from build123d import *

# Parameters (mm, degrees)
SKETCH1_W                 = 12
SKETCH1_H                 = 25
BOSS_EXTRUDE1_DEPTH       = 16
SKETCH2_W                 = 32
SKETCH2_H                 = 10
BOSS_EXTRUDE2_DEPTH       = 16.2
BOSS_EXTRUDE3_DEPTH       = 32
M5X0_8_TAPPED_HOLE1_D     = 4.2
M5X0_8_TAPPED_HOLE1_DEPTH = 9
M5X0_8_TAPPED_HOLE1_TIP   = 1.2618073
CUT_EXTRUDE2_REACH        = 27
M3X0_5_TAPPED_HOLE1_D     = 2.75
M3X0_5_TAPPED_HOLE1_DEPTH = 12
M3X0_5_TAPPED_HOLE1_TIP   = 0.826183351


with BuildPart() as part:
    # Sketch1 → Boss-Extrude1 (new body, symmetric)
    with BuildSketch(Plane(origin=(0, 0, 0), x_dir=(0, 0, -1), z_dir=(1, 0, 0))):
        with Locations((6, 12.5)):
            Rectangle(SKETCH1_W, SKETCH1_H)
    extrude(amount=BOSS_EXTRUDE1_DEPTH, both=True)



with BuildPart() as body_2:
    # Sketch2 → Boss-Extrude2 (new body)
    with BuildSketch(Plane(origin=(0, 0, 0), x_dir=(1, 0, 0), z_dir=(0, 1, 0))):
        with Locations((0, -7)):
            Rectangle(SKETCH2_W, SKETCH2_H)
    extrude(amount=BOSS_EXTRUDE2_DEPTH)


with BuildPart() as part_1:
    add(part.part)

    add(body_2.part)  # Boss-Extrude3 merges body 2
    # Sketch3 → Boss-Extrude3 (add)
    with BuildSketch(Plane(origin=(16, 0, 0), x_dir=(0, 0, -1), z_dir=(1, 0, 0))):
        Polygon((-2, 0), (-2, 16.2), (0, 25), (0, 0), align=None)
    extrude(amount=-BOSS_EXTRUDE3_DEPTH)

    # M5x0.8 Tapped Hole1
    with Locations(Plane(origin=(0, 0, -12), x_dir=(-1, 0, 0), z_dir=(0, 0, -1))):
        with Locations((0, 20), (0, 5)):
            Hole(M5X0_8_TAPPED_HOLE1_D / 2, depth=M5X0_8_TAPPED_HOLE1_DEPTH)
            with Locations((0, 0, -(M5X0_8_TAPPED_HOLE1_DEPTH + M5X0_8_TAPPED_HOLE1_TIP / 2))):  # 118° drill point
                Cone(0, M5X0_8_TAPPED_HOLE1_D / 2, M5X0_8_TAPPED_HOLE1_TIP, mode=Mode.SUBTRACT)

    # Sketch9 → Cut-Revolve1 (revolve, cut)
    with BuildSketch(Plane(origin=(0, 0, 0), x_dir=(0, 0, -1), z_dir=(1, 0, 0))):
        Polygon((-12, 16.2), (-4, 16.2), (-4, 12), (-6, 12), (-6, 6.5), (-4, 6.5), (-4, 0), (-12, 0), align=None)
    revolve(axis=Axis((0, 0, 12), (0, 1, 0)), mode=Mode.SUBTRACT)

    # Sketch10 → Cut-Extrude2 (cut, up to next)
    with BuildSketch(Plane(origin=(0, 25, 0), x_dir=(1, 0, 0), z_dir=(0, 1, 0)), mode=Mode.PRIVATE) as cut_extrude2_sk1:
        Polygon((6.3625, 12), (14.623214286, 0), (16, 0), (16, 12), align=None)
    cut_extrude2_tool1 = extrude(cut_extrude2_sk1.sketch, amount=-CUT_EXTRUDE2_REACH, mode=Mode.PRIVATE) & part_1.part
    add(cut_extrude2_tool1.solids().sort_by_distance((12.730134, 25, -7.5))[0], mode=Mode.SUBTRACT)
    # Sketch10 → Cut-Extrude2 (cut, up to next)
    with BuildSketch(Plane(origin=(0, 25, 0), x_dir=(1, 0, 0), z_dir=(0, 1, 0)), mode=Mode.PRIVATE) as cut_extrude2_sk2:
        Polygon((16, 0), (14.623214286, 0), (16, -2), align=None)
    cut_extrude2_tool2 = extrude(cut_extrude2_sk2.sketch, amount=-CUT_EXTRUDE2_REACH, mode=Mode.PRIVATE) & part_1.part
    add(cut_extrude2_tool2.solids().sort_by_distance((15.541071, 25, 0.666667))[0], mode=Mode.SUBTRACT)
    # Sketch10 → Cut-Extrude2 (cut, up to next)
    with BuildSketch(Plane(origin=(0, 25, 0), x_dir=(1, 0, 0), z_dir=(0, 1, 0)), mode=Mode.PRIVATE) as cut_extrude2_sk3:
        Polygon((-16, 0), (-14.623214286, 0), (-6.3625, 12), (-16, 12), align=None)
    cut_extrude2_tool3 = extrude(cut_extrude2_sk3.sketch, amount=-CUT_EXTRUDE2_REACH, mode=Mode.PRIVATE) & part_1.part
    add(cut_extrude2_tool3.solids().sort_by_distance((-12.730134, 25, -7.5))[0], mode=Mode.SUBTRACT)
    # Sketch10 → Cut-Extrude2 (cut, up to next)
    with BuildSketch(Plane(origin=(0, 25, 0), x_dir=(1, 0, 0), z_dir=(0, 1, 0)), mode=Mode.PRIVATE) as cut_extrude2_sk4:
        Polygon((-16, 0), (-16, -2), (-14.623214286, 0), align=None)
    cut_extrude2_tool4 = extrude(cut_extrude2_sk4.sketch, amount=-CUT_EXTRUDE2_REACH, mode=Mode.PRIVATE) & part_1.part
    add(cut_extrude2_tool4.solids().sort_by_distance((-15.541071, 25, 0.666667))[0], mode=Mode.SUBTRACT)

    # M3x0.5 Tapped Hole1
    with Locations(Plane.XY.offset(12)):
        with Locations((-11.5, 13.25), (11.5, 13.25), (-11.5, 5.25), (11.5, 5.25)):
            Hole(M3X0_5_TAPPED_HOLE1_D / 2, depth=M3X0_5_TAPPED_HOLE1_DEPTH)
            with Locations((0, 0, -(M3X0_5_TAPPED_HOLE1_DEPTH + M3X0_5_TAPPED_HOLE1_TIP / 2))):  # 118° drill point
                Cone(0, M3X0_5_TAPPED_HOLE1_D / 2, M3X0_5_TAPPED_HOLE1_TIP, mode=Mode.SUBTRACT)


solid = part_1.part
Model file for the job. Use its own axes, mm. A direction names the side the tool comes from. Give positions to 0.01 mm unless a question says otherwise; leave off trailing zeros. Loops run counter-clockwise (first coordinate to the right, second up) from the corner with the lowest first, then second, coordinate; pieces in that order, holes last. Notation, with made-up numbers: (81, 82.5) -> (109, 82.5) arc R22 cw to (109, 121.5) -> close; hole circle Ø11 at (67.25, -24). An arc over 180 degrees is marked (long way). Use a Markdown table: item, result. Add a question column.
(1) Slice it at D-D on x = -14. List the corners of the cut face in (y, z), and give its area (3 significant figures).
(2) Slice it at A-A on z = 3.25. List the corners of the cut face in (x, y) (3 decimals).
(3) Mould opens along Y. For faces 4 (the flat face through (12, 8, 12)), 5 (the flat face through (0.6, 12, 5.6)), 6 (the conical face through (-0.2, 5.31, -1.96)) say: +Y half, -Y half, draft (parallel to the pull), parting line (faces both ways), or undercut.
(4) Slice it at B-B on z = 7.75. List the corners of the cut face in (x, y) (3 decimals), and give its area (3 significant figures).
(5) Slice it at C-C on y = 9.25. List the corners of the cut face in (x, z), and give its area (3 significant figures).
(6) Drop flat-ended pins along their axis: pin 1 Ø2 at (x, y) = (-11.5, 13.25) entering from +Z; pin 2 Ø4 at (x, z) = (-2.5, 8.5) entering from -Y; pin 3 Ø10 at (x, z) = (12, 7.5) entering from -Y; pin 4 Ø2 at (x, y) = (11.5, 13.25) entering from -Z. Give the stop position or say it passes through.
(7) Tool access for faces 1 (the cylindrical face through (12.874, 5.31, 5.916)), 2 (the flat face through (0, 6.5, 5)), 3 (the flat face through (-0.2, 16.2, 3.6)): list every direction of +Z, -Z, +X, -X, +Y, -Y with a clear straight run to the whole face (end or side of a thin tool).
(8) Wall check: line 1 along Y through (x, z) = (11.5, 6.75) (3 decimals); line 2 along Y through (x, z) = (0, -5.5); line 3 along X through (y, z) = (5.25, 7.5) (3 decimals). Give the ranges that are in metal, low to high.
Filled sheet:
| question | item | result |
|---|---|---|
| 1 | outline | (0, -0.91) -> (25, -0.91) -> (25, 0) -> (16.2, 2) -> (16.2, 12) -> (0, 12) -> close |
| 1 | area | 226 mm2 |
| 2 | outline | (-16, 0) -> (16, 0) -> (16, 16.2) -> (-16, 16.2) -> close; hole circle Ø2.75 at (-11.5, 5.25); hole circle Ø2.75 at (-11.5, 13.25); hole circle Ø2.75 at (11.5, 5.25); hole circle Ø2.75 at (11.5, 13.25) |
| 3 | face 4 | draft |
| 3 | face 5 | +Y half |
| 3 | face 6 | undercut |
| 4 | outline | (-16, 0) -> (-6.778, 0) -> (-6.778, 6.5) -> (-4.235, 6.5) -> (-4.235, 12) -> (-6.778, 12) -> (-6.778, 16.2) -> (-16, 16.2) -> close; (4.235, 6.5) -> (6.778, 6.5) -> (6.778, 0) -> (16, 0) -> (16, 16.2) -> (6.778, 16.2) -> (6.778, 12) -> (4.235, 12) -> close; hole circle Ø2.75 at (-11.5, 5.25); hole circle Ø2.75 at (-11.5, 13.25); hole circle Ø2.75 at (11.5, 5.25); hole circle Ø2.75 at (11.5, 13.25) |
| 4 | area | 303 mm2 |
| 5 | outline | (-16, 2) -> (-6.36, -12) -> (6.36, -12) -> (16, 2) -> (16, 12) -> (6, 12) arc R6 cw to (-6, 12) -> (-16, 12) -> close |
| 5 | area | 577 mm2 |
| 6 | pin 1 | z = -0.23 |
| 6 | pin 2 | y = 6.5 |
| 6 | pin 3 | y = 0 |
| 6 | pin 4 | z = -5.99 |
| 7 | face 1 | +Z |
| 7 | face 2 | +Z, -Y |
| 7 | face 3 | +Z, +X, -X, +Y |
| 8 | line 1 | 0 to 3.875, 6.625 to 11.875, 14.625 to 16.2 |
| 8 | line 2 | 0 to 2.9, 7.1 to 17.9, 22.1 to 25 |
| 8 | line 3 | -16 to -12.875, -10.125 to -6.614, 6.614 to 10.125, 12.875 to 16 |
